```python
from build123d import *

# Parameters (mm, degrees)
BOSS_EXTRUDE1_DEPTH     = 25
CUT_EXTRUDE1_DEPTH      = 1
CUT_EXTRUDE1_DEPTH_BACK = 51


with BuildPart() as part:
    # Sketch4 → Boss-Extrude1 (new body, symmetric)
    with BuildSketch(Plane.XY):
        with BuildLine():
            Line((0, -5.45), (0.655464476, -6))
            Line((0.655464476, -6), (4.504469158, -6))
            Line((4.504469158, -6), (8.25, -9.745530842))
            Line((8.25, -9.745530842), (8.25, -12.885))
            Line((8.25, -12.885), (4, -12.885))
            Line((4, -12.885), (4, -14.45))
            Line((4, -14.45), (4.55, -14.45))
            Line((4.55, -14.45), (4.55, -15))
            Line((4.55, -15), (12.885, -15))
            ThreePointArc((12.885, -15), (14.380530842, -14.380530842), (15, -12.885))
            Line((15, -12.885), (15, -4.55))
            Line((15, -4.55), (14.45, -4.55))
            Line((14.45, -4.55), (14.45, -4))
            Line((14.45, -4), (12.885, -4))
            Line((12.885, -4), (12.885, -8.25))
            Line((12.885, -8.25), (9.745530842, -8.25))
            Line((9.745530842, -8.25), (6, -4.504469158))
            Line((6, -4.504469158), (6, -0.655464476))
            Line((6, -0.655464476), (5.45, 0))
            Line((5.45, 0), (3.5, 0))
            ThreePointArc((3.5, 0), (3.371433308, -0.939913534), (2.995178599, -1.81077474))
            Line((2.995178599, -1.81077474), (4.675743591, -3.491339732))
            Line((4.675743591, -3.491339732), (3.491339732, -4.675743591))
            Line((3.491339732, -4.675743591), (1.81077474, -2.995178599))
            ThreePointArc((1.81077474, -2.995178599), (0.939913534, -3.371433308), (0, -3.5))
            Line((0, -3.5), (0, -5.45))
        make_face()
        with BuildLine():
            Line((9.375, -10.365), (9.375, -12.885))
            ThreePointArc((9.375, -12.885), (9.664964287, -13.585035713), (10.365, -13.875))
            Line((10.365, -13.875), (12.885, -13.875))
            ThreePointArc((12.885, -13.875), (13.585035713, -13.585035713), (13.875, -12.885))
            Line((13.875, -12.885), (13.875, -10.365))
            ThreePointArc((13.875, -10.365), (13.585035713, -9.664964287), (12.885, -9.375))
            Line((12.885, -9.375), (10.365, -9.375))
            ThreePointArc((10.365, -9.375), (9.664964287, -9.664964287), (9.375, -10.365))
        make_face(mode=Mode.SUBTRACT)
    extrude(amount=BOSS_EXTRUDE1_DEPTH, both=True)

    # Mirror1: part across plane


with BuildPart() as part_1:
    add(part.part)
    add(part.part.mirror(Plane(origin=(0, 0, 0), x_dir=(0, 0, 1), z_dir=(1, 0, 0))))

    # Mirror2: part across plane


with BuildPart() as part_2:
    add(part_1.part)
    add(part_1.part.mirror(Plane.ZX))

    # Sketch5 → Cut-Extrude1 (cut, two sides)
    with BuildSketch(Plane.XY.offset(25)) as cut_extrude1_sk:
        Polygon((-5.675, 12.885), (-5.4, 13.16), (-5.125, 12.885), align=None)
    extrude(amount=CUT_EXTRUDE1_DEPTH, mode=Mode.SUBTRACT)
    extrude(cut_extrude1_sk.sketch, amount=-CUT_EXTRUDE1_DEPTH_BACK, mode=Mode.SUBTRACT)


solid = part_2.part
```
Could you check a few things on this model? Use its own coordinates, in mm. A direction names the side the tool comes from. Round coordinates to 2 decimals unless told otherwise and drop trailing zeros. Loops run counter-clockwise (first coordinate to the right, second up) from the corner with the lowest first, then second, coordinate; pieces in that order, holes last.
Q1. Please list where these lines run through material, in increasing order: L1, parallel to Y at x = 10.25, z = 22; L2, parallel to Y at x = 13, z = -5; L3, parallel to X at y = 4.5, z = 22 (3 decimals).
Q2. On a 3-axis mill with a long thin cutter (end or side, diameter ignored), from which of +Z, -Z, +X, -X, +Y, -Y can I reach the whole of each face in a straight line? I mean faces 1 (the cylindrical face through (9.67, -9.66, 0.35)), 2 (the flat face through (15, -9, 0)), 3 (the flat face through (14, 4, 0)). Say none if no direction works.
Q3. I want a section at D-D (z = -15). Give the number of separate pieces and of enclosed holes in the cut face, and give its area (3 significant figures).
Q4. I want a section at C-C (y = -1.25). Write out the boundary of the cut face in (x, z).
Q5. I want a section at A-A (y = -11.5). Write out the boundary of the cut face in (x, z) (3 decimals).
Q6. For P1, Ø1, axis at x = -3, z = -5.5, coming from the -Y side; P2, Ø0.6, axis at y = -14.5, z = -9.5, coming from the -X side; P3, Ø1.5, axis at x = -3, y = -10.5, coming from the -Z side; P4, Ø1.7, axis at y = 14, z = 4.5, coming from the +X side, each with a flat end and sliding along its axis, tell me the tip position at first contact or that it passes through.
Answer below:
1. L1: y = -15 to -13.87, -9.38 to -8.25, 8.25 to 9.38, 13.87 to 15
1. L2: y = -15 to -13.87, -9.38 to -4, 4 to 9.38, 13.87 to 15
1. L3: x = -14.45 to -12.885, -6 to -3.667, -3.316 to 3.316, 3.667 to 6, 12.885 to 14.45
2. face 1: +Z, -Z
2. face 2: +Z, -Z, +X, +Y, -Y
2. face 3: +Z, -Z, +X
3. separate pieces: 1
3. enclosed holes: 5
3. area: 295 mm2
4. outline: (-6, -25) - (-3.27, -25) - (-3.27, 25) - (-6, 25) - close; (3.27, -25) - (6, -25) - (6, 25) - (3.27, 25) - close
5. outline: (-15, -25) - (-13.875, -25) - (-13.875, 25) - (-15, 25) - close; (-9.375, -25) - (-8.25, -25) - (-8.25, 25) - (-9.375, 25) - close; (8.25, -25) - (9.375, -25) - (9.375, 25) - (8.25, 25) - close; (13.875, -25) - (15, -25) - (15, 25) - (13.875, 25) - close
6. P1: stops at y = -6
6. P2: stops at x = -14.54
6. P3: passes through
6. P4: stops at x = 14.98
